from build123d import *

# Parameters (mm, degrees)
SALIENTE_EXTRUIR1_DEPTH = 30
CROQUIS2_W              = 18
CROQUIS2_H              = 35
CORTAR_EXTRUIR1_DEPTH   = 99.107084352
CROQUIS3_R              = 20
SALIENTE_EXTRUIR3_DEPTH = 22
CROQUIS3_4_R            = 8
CORTAR_EXTRUIR2_DEPTH   = 22
CROQUIS4_W              = 24
CROQUIS4_H              = 11.9
CORTAR_EXTRUIR6_DEPTH   = 20


with BuildPart() as part:
    # Croquis1 → Saliente-Extruir1 (new, symmetric)
    with BuildSketch(Plane(origin=(0, 0, 0), x_dir=(0, 0, -1), z_dir=(1, 0, 0))):
        Polygon((45, -25), (-45, -25), (-25, 25), (25, 25), align=None)
    extrude(amount=SALIENTE_EXTRUIR1_DEPTH, both=True)

    # Croquis2 → Cortar-Extruir1 (cut, through all)
    with BuildSketch(Plane.XY.offset(45)):
        with Locations((-21, 7.5)):
            Rectangle(CROQUIS2_W, CROQUIS2_H)
        with Locations((21, 7.5)):
            Rectangle(CROQUIS2_W, CROQUIS2_H)
    extrude(amount=-CORTAR_EXTRUIR1_DEPTH, mode=Mode.SUBTRACT)

    # Croquis3 → Saliente-Extruir3 (add, symmetric)
    with BuildSketch(Plane(origin=(0, 0, 0), x_dir=(0, 0, -1), z_dir=(1, 0, 0))):
        with Locations((0, 25)):
            Circle(CROQUIS3_R)
    extrude(amount=SALIENTE_EXTRUIR3_DEPTH, both=True)

    # Croquis3<4> → Cortar-Extruir2 (cut, symmetric)
    with BuildSketch(Plane(origin=(0, 0, 0), x_dir=(0, 0, -1), z_dir=(1, 0, 0))):
        with Locations((0, 25)):
            Circle(CROQUIS3_4_R)
    extrude(amount=CORTAR_EXTRUIR2_DEPTH, both=True, mode=Mode.SUBTRACT)

    # Croquis4 → Cortar-Extruir6 (cut)
    with BuildSketch(Plane(origin=(0, 45, 0), x_dir=(1, 0, 0), z_dir=(0, 1, 0))):
        with Locations((0, 14.05)):
            Rectangle(CROQUIS4_W, CROQUIS4_H)
        with Locations((0, -14.05)):
            Rectangle(CROQUIS4_W, CROQUIS4_H)
    extrude(amount=-CORTAR_EXTRUIR6_DEPTH, mode=Mode.SUBTRACT)


solid = part.part
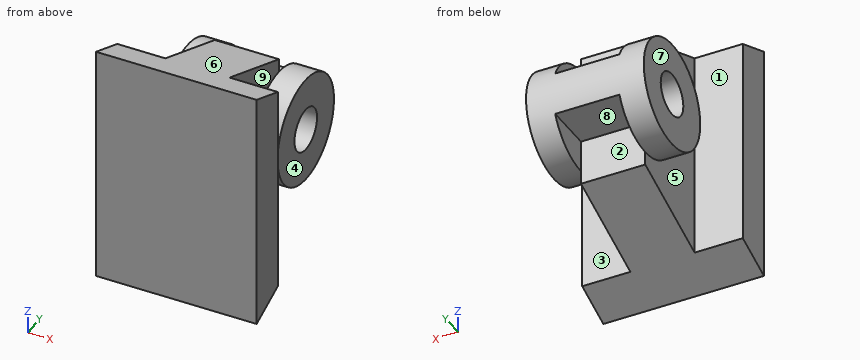
Input: part model. Units: mm. Frame: model coordinates. Face numbers are marked on the shaded views. A direction names the side the tool comes from. Coordinates: 2 decimals unless noted, no trailing zeros. Loops run counter-clockwise (first coordinate to the right, second up) from the corner with the lowest first, then second, coordinate; pieces in that order, holes last.
Q1. Set-up query: the marked faces 1, 2, 3, 4 and 5. Return all of +Z, -Z, +X, -X, +Y, -Y with unobstructed straight access to the full face (end or side cutting, diameter ignored); none if empty.
Q2. Cut plane B-B (z = 0). Output: boundary loops of the cut face in (x, y), then the cut area to 3 significant figures.
Q3. Material intervals for line 1 (Y direction, x = 3.5, z = 0); line 2 (Y direction, x = -2, z = -12.5); line 3 (X direction, y = 0, z = -28), sorted ascending.
Q4. Cut plane D-D (z = 28). Output: boundary loops of the cut face in (x, y).
Q5. Draft query along X for the marked faces 6, 7, 8 and 9. Return one class per face: +X half, -X half, draft (parallel to the pull), parting line (faces both ways), or undercut.
Q6. Cut plane A-A (x = 9). Output: boundary loops of the cut face in (y, z).
Q7. Contact query for flat-ended pins moving along their axis: pin 1 (1 mm diameter, centred on x = 15, y = 7.5, fed in from -Z); pin 2 (20 mm diameter, centred on x = -2.5, y = 30, fed in from +Z); pin 3 (3 mm diameter, centred on x = 2, y = 26, fed in from -Z); pin 4 (8 mm diameter, centred on y = 18, z = -32.5, fed in from +X). Output: stop coordinate, or through.
Q8. Cut plane C-C (y = 31.5). Output: boundary loops of the cut face in (x, z), then the cut area to 3 significant figures.
Working result:
1. face 1: +Z, -Z, -X
1. face 2: -Z, +Y
1. face 3: +Z, -Z, +X
1. face 4: +Z, -Z, +X, +Y
1. face 5: -X
2. outline: (-30, -25) - (30, -25) - (30, -10) - (12, -10) - (12, 5) - (22, 5) - (22, 17) - (-22, 17) - (-22, 5) - (-12, 5) - (-12, -10) - (-30, -10) - close; (-22, 33) - (22, 33) - (22, 45) - (-22, 45) - close
2. area: 2,320 mm2
3. line 1: y = -25 to 17, 33 to 45
3. line 2: y = -25 to 25
3. line 3: x = -12 to 12
4. outline: (-30, -25) - (30, -25) - (30, -10) - (12, -10) - (12, 17.5) - (-12, 17.5) - (-12, -10) - (-30, -10) - close
5. face 6: draft
5. face 7: -X half
5. face 8: undercut
5. face 9: +X half
6. outline: (-25, -45) - (25, -25) - (25, -8.1) - (43.29, -8.1) arc R20 ccw to (43.29, 8.1) - (25, 8.1) - (25, 25) - (-25, 45) - close; hole circle Ø16 at (25, 0)
7. pin 1: stops at z = -10.54
7. pin 2: stops at z = 27
7. pin 3: stops at z = -25.2
7. pin 4: passes through
8. outline: (-22, -18.91) - (-12, -18.91) - (-12, -8.1) - (12, -8.1) - (12, -18.91) - (22, -18.91) - (22, -4.66) - (-22, -4.66) - close; (-22, 4.66) - (22, 4.66) - (22, 18.91) - (12, 18.91) - (12, 8.1) - (-12, 8.1) - (-12, 18.91) - (-22, 18.91) - close
8. area: 735 mm2
